Source: CAD feature listing. Evaluate the final solid. Frame: model axes, mm. Face numbers are marked on the shaded views. A direction names the side the tool comes from. Give positions to 0.01 mm unless a question says otherwise; leave off trailing zeros. Write each loop counter-clockwise with the first axis right and the second up, starting at its lowest first coordinate (ties: lowest second). Pieces come first, ordered by that corner, then holes.
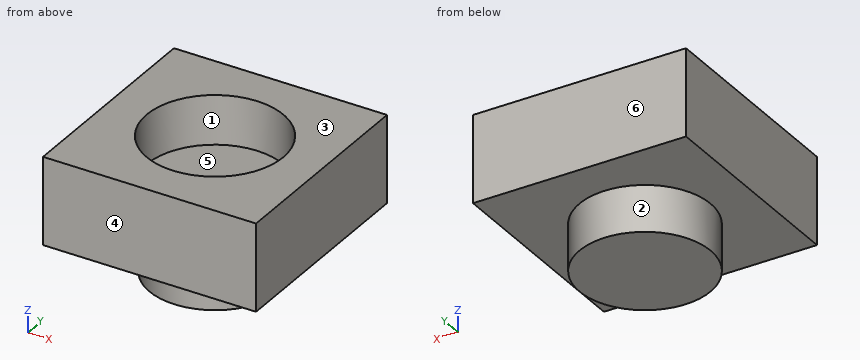
```python
from build123d import *

# Parameters (mm, degrees)
SKETCH_1_W          = 7.8
SKETCH_1_H          = 7.8
EXTRUDE_1_DEPTH     = 3.2
SKETCH_2_R          = 2.5
CUT_EXTRUDE_1_DEPTH = 1.8
SKETCH_3_R          = 2.4
EXTRUDE_2_DEPTH     = 1.7


with BuildPart() as part:
    # Эскиз1 → Бобышка-Вытянуть1 (new body)
    with BuildSketch(Plane.XY):
        Rectangle(SKETCH_1_W, SKETCH_1_H)
    extrude(amount=EXTRUDE_1_DEPTH)

    # Эскиз2 → Вырез-Вытянуть1 (cut)
    with BuildSketch(Plane.XY.offset(3.2)):
        Circle(SKETCH_2_R)
    extrude(amount=-CUT_EXTRUDE_1_DEPTH, mode=Mode.SUBTRACT)

    # Эскиз3 → Бобышка-Вытянуть2 (add)
    with BuildSketch(Plane(origin=(0, 0, 0), x_dir=(-1, 0, 0), z_dir=(0, 0, -1))):
        Circle(SKETCH_3_R)
    extrude(amount=EXTRUDE_2_DEPTH)


solid = part.part
```
1. Line query: probe 1 along Y at (x, z) = (0, 2.85); probe 2 along Z at (x, y) = (-1.5, -1); probe 3 along Z at (x, y) = (2.5, -1.75). Output: solid intervals per line, ascending.
2. Section query D-D (y = 3.5). Return loops of the section in (x, z), plus the area to 3 significant figures.
3. Pull-direction query (Y, two-part tool) for the marked faces 4, 5 and 6; classes: pulls with the +Y half, pulls with the -Y half, needs draft (parallel to the pull), parting line crosses it, or undercut.
4. Access query for the marked faces 1, 2 and 3. Directions: +Z, -Z, +X, -X, +Y, -Y. A direction counts if a zero-diameter tool reaches every point of the face in a straight line with its end or side. Return the directions, or none.
5. Pin query (flat end, axial travel): P1, Ø4, axis at x = -0.5, y = -1, coming from the +Z side; P2, Ø4.5, axis at x = 0, y = 0, coming from the +Z side. Return the tip coordinate at first contact, or that it passes through.
6. Section query C-C (z = -0.35). Return loops of the section in (x, y), plus the area to 3 significant figures.
7. Section query A-A (x = 0). Return loops of the section in (y, z).
The answers:
1. probe 1: y = -3.9 to -2.5, 2.5 to 3.9
1. probe 2: z = -1.7 to 1.4
1. probe 3: z = 0 to 3.2
2. outline: (-3.9, 0) - (3.9, 0) - (3.9, 3.2) - (-3.9, 3.2) - close
2. area: 25.0 mm2
3. face 4: pulls with the -Y half
3. face 5: undercut
3. face 6: pulls with the +Y half
4. face 1: +Z
4. face 2: -Z
4. face 3: +Z, +X, -X, +Y, -Y
5. P1: stops at z = 3.2
5. P2: stops at z = 1.4
6. outline: circle Ø4.8 at (0, 0)
6. area: 18.1 mm2
7. outline: (-3.9, 0) - (-2.4, 0) - (-2.4, -1.7) - (2.4, -1.7) - (2.4, 0) - (3.9, 0) - (3.9, 3.2) - (2.5, 3.2) - (2.5, 1.4) - (-2.5, 1.4) - (-2.5, 3.2) - (-3.9, 3.2) - close
